```python
from build123d import *

# Parameters (mm, degrees)
F0_W     = 974
F0_H     = 224
F0_H_2   = 237
F1_DEPTH = 300


with BuildPart() as f1:
    # F0 (on Top) → F1 (new body)
    with BuildSketch(Plane.XY):
        Polygon((0, 13), (0, 0), (1000, 0), (1000, 13), (1000, 237), (1000, 250), (1000, 500), (1000, 750), (1000, 1000), (0, 1000), (0, 750), (0, 500), (0, 250), (0, 237), align=None)
        with Locations((500, 125)):
            Rectangle(F0_W, F0_H, mode=Mode.SUBTRACT)
        with Locations((500, 368.5)):
            Rectangle(F0_W, F0_H_2, mode=Mode.SUBTRACT)
        with Locations((500, 618.5)):
            Rectangle(F0_W, F0_H_2, mode=Mode.SUBTRACT)
        with Locations((500, 868.5)):
            Rectangle(F0_W, F0_H_2, mode=Mode.SUBTRACT)
    extrude(amount=F1_DEPTH)


solid = f1.part
```
The model under review builds one solid part; all positions refer to its coordinate system, in mm. A direction names the side the tool comes from. Give positions to 0.01 mm unless a question says otherwise; leave off trailing zeros. Write each loop counter-clockwise with the first axis right and the second up, starting at its lowest first coordinate (ties: lowest second). Pieces come first, ordered by that corner, then holes. Notation, with made-up numbers: (-35.75, 11) - (6.25, 11) arc R29 ccw to (6.25, 39) - close; hole circle Ø2 at (4.25, 26.5). An arc over 180 degrees is marked (long way). Answer in a Markdown table with one row per item. Add a question column.
1. We need section A-A on y = 427. Write out the cut boundary in (x, z).
2. We need section B-B on x = 890.5. Write out the cut boundary in (y, z), then the cut area to 3 significant figures.
3. Tool access review of faces 4 (the flat face through (1000, 493, 148)), 5 (the flat face through (13, 617, 148)): name each direction out of +Z, -Z, +X, -X, +Y, -Y from which nothing blocks a thin tool from reaching the whole face with its end or side.
4. Insertion check: P1, Ø8, axis at y = 440, z = 136, coming from the -X side. The pin has a flat end and moves straight along its axis. Give the tip position at first contact, or say it passes through.
5. Wall thickness on line 1 along Y through (x, z) = (665, 31); line 2 along X through (y, z) = (174.5, 257): over which ranges is each line inside the solid? List them lowest first. Write a range as [from, to].
6. Draft analysis for pull direction Y (two halves, no side actions). For faces 1 (the flat face through (498, 243, 300)), 2 (the flat face through (493, 13, 148)), 3 (the flat face through (507, 1000, 148)), state which applies: +Y half, -Y half, draft (parallel to the pull), parting line (faces both ways), or undercut.
7. We need section C-C on z = 158. Write out the cut boundary in (x, y).
Ans:
| question | item | result |
|---|---|---|
| 1 | outline | (0, 0) - (13, 0) - (13, 300) - (0, 300) - close; (987, 0) - (1000, 0) - (1000, 300) - (987, 300) - close |
| 2 | outline | (0, 0) - (13, 0) - (13, 300) - (0, 300) - close; (237, 0) - (250, 0) - (250, 300) - (237, 300) - close; (487, 0) - (500, 0) - (500, 300) - (487, 300) - close; (737, 0) - (750, 0) - (750, 300) - (737, 300) - close; (987, 0) - (1000, 0) - (1000, 300) - (987, 300) - close |
| 2 | area | 19,500 mm^2 |
| 3 | face 4 | +Z, -Z, +X, +Y, -Y |
| 3 | face 5 | +Z, -Z |
| 4 | P1 | stops at x = 0 |
| 5 | line 1 | y = [0, 13], [237, 250], [487, 500], [737, 750], [987, 1000] |
| 5 | line 2 | x = [0, 13], [987, 1000] |
| 6 | face 1 | draft |
| 6 | face 2 | undercut |
| 6 | face 3 | +Y half |
| 7 | outline | (0, 0) - (1000, 0) - (1000, 1000) - (0, 1000) - close; hole (13, 13) - (987, 13) - (987, 237) - (13, 237) - close; hole (13, 250) - (987, 250) - (987, 487) - (13, 487) - close; hole (13, 500) - (987, 500) - (987, 737) - (13, 737) - close; hole (13, 750) - (987, 750) - (987, 987) - (13, 987) - close |
